Autodesk Inventor part; units mm, degrees
ref_plane "YZ Plane" through (0, 0, 0) normal (1, 0, 0) x (0, 1, 0)
ref_plane "XZ Plane" through (0, 0, 0) normal (0, 1, 0) x (-1, 0, 0)
ref_plane "XY Plane" through (0, 0, 0) normal (0, 0, 1) x (1, 0, 0)
sketch "草圖1" plane through (0, 0, 0) normal (0, 1, 0) x (-1, 0, 0)
  line L0 (0, 0) -> (60, 0)
  line L1 (60, 0) -> (60, -90)
  line L2 (60, -90) -> (0, -90)
  line L3 (0, -90) -> (0, 0)
  dimension "d0" = 60
  dimension "d1" = 90
extrude "擠出1" add sketch "草圖1" along normal blind 10
chamfer "倒角1" distance 5 angle 45 4 edges at (-60, 10, -45) (-30, 10, 0) (0, 10, -45) (-30, 10, -90)
sketch "草圖2" plane through (0, 10, 0) normal (0, 1, 0) x (1, 0, 0)
  line L0 (-60, 0) -> (0, 0)
  line L1 (0, 0) -> (-15, 0)
  line L2 (-15, 0) -> (-15, 10)
  line L3 (-15, 10) -> (0, 10)
  line L4 (0, 10) -> (0, 0)
  line L5 (-15, 10) -> (-30, 10)
  line L6 (-30, 10) -> (-30, 15)
  line L7 (-30, 15) -> (-15, 15)
  line L8 (-15, 15) -> (-15, 10)
  line L9 (-30, 15) -> (-35, 15)
  line L10 (-35, 15) -> (-35, 35)
  line L11 (-35, 35) -> (-30, 35)
  line L12 (-30, 35) -> (-30, 15)
  line L13 (-35, 35) -> (-50, 35)
  line L14 (-50, 35) -> (-50, 80)
  line L15 (-50, 80) -> (-35, 80)
  line L16 (-35, 80) -> (-35, 35)
  line L17 (-35, 80) -> (-20, 80)
  line L18 (-20, 80) -> (-20, 75)
  line L19 (-20, 75) -> (-35, 75)
  line L20 (-35, 75) -> (-35, 80)
  line L21 (-20, 75) -> (-10, 75)
  line L22 (-10, 75) -> (-10, 45)
  line L23 (-10, 45) -> (-20, 45)
  line L24 (-20, 45) -> (-20, 75)
  circle A0 centre (-15, 10) radius 3
  circle A1 centre (-30, 15) radius 3
  circle A2 centre (-35, 35) radius 3
  circle A3 centre (-50, 80) radius 3
  circle A4 centre (-20, 75) radius 3
  circle A5 centre (-10, 45) radius 3
  dimension "d7" = 15
  dimension "d8" = 10
  dimension "d9" = 15
  dimension "d10" = 5
  dimension "d11" = 5
  dimension "d12" = 20
  dimension "d13" = 15
  dimension "d14" = 45
  dimension "d15" = 15
  dimension "d16" = 5
  dimension "d17" = 10
  dimension "d18" = 30
  dimension "d19" = 6
  dimension "d20" = 6
  dimension "d21" = 6
  dimension "d22" = 6
  dimension "d23" = 6
  dimension "d24" = 6
extrude "擠出2" add sketch "草圖2" along normal blind 40 contours A5 L22 L23 | L23 L22 A5
extrude "擠出3" add sketch "草圖2" along normal blind 5 contours A4 L18 L19 | L19 L24 A4 | L18 A4 L21 | L21 A4 L24
extrude "擠出4" add sketch "草圖2" along normal blind 10 contours A3 L15 L14 | L14 L15 A3
extrude "擠出5" add sketch "草圖2" along normal blind 25 contours A2 L13 L10 | L10 L11 A2 | L11 L16 A2 | L13 A2 L16
extrude "擠出6" add sketch "草圖2" along normal blind 20 contours A0 L5 L2 | L2 L3 A0 | L8 A0 L3 | L5 A0 L8
extrude "擠出7" add sketch "草圖2" along normal blind 30 contours A1 L9 L6 | L6 L7 A1 | L7 L12 A1 | L9 A1 L12
sketch "草圖3" plane through (-15, 30, -10) normal (0, 1, 0) x (1, 0, 0)
  circle A0 centre (0, 0) radius 1.5
  point P0 (15, -10)
  dimension "d37" = 3
sketch "草圖4" plane through (-30, 40, -15) normal (0, 1, 0) x (1, 0, 0)
  circle A0 centre (0, 0) radius 1.5
  point P0 (30, -15)
  dimension "d38" = 3
sketch "草圖5" plane through (-10, 50, -45) normal (0, 1, 0) x (1, 0, 0)
  circle A0 centre (0, 0) radius 1.5
  point P0 (10, -45)
  dimension "d39" = 3
sketch "草圖6" plane through (-35, 35, -35) normal (0, 1, 0) x (1, 0, 0)
  circle A0 centre (0, 0) radius 1.5
  point P0 (35, -35)
  dimension "d40" = 3
sketch "草圖7" plane through (-50, 20, -80) normal (0, 1, 0) x (1, 0, 0)
  circle A0 centre (0, 0) radius 1.5
  point P0 (50, -80)
  dimension "d41" = 3
sketch "草圖8" plane through (-20, 15, -75) normal (0, 1, 0) x (1, 0, 0)
  circle A0 centre (0, 0) radius 1.5
  point P0 (20, -75)
  dimension "d42" = 3
extrude "擠出8" add sketch "草圖8" along normal blind 8
extrude "擠出9" add sketch "草圖5" along normal blind 8
extrude "擠出10" add sketch "草圖3" along normal blind 8
extrude "擠出11" add sketch "草圖4" along normal blind 8
extrude "擠出12" add sketch "草圖6" along normal blind 8
extrude "擠出13" add sketch "草圖7" along normal blind 8
chamfer "倒角2" distance 0.5 distance2 8 1 edges at (-51.5, 28, -80) measured on face at (-50.167, 28, -80.5524)
chamfer "倒角3" distance 0.5 distance2 8 1 edges at (-21.5, 23, -75) measured on face at (-20.167, 23, -75.5524)
chamfer "倒角4" distance 0.5 distance2 8 1 edges at (-11.5, 58, -45) measured on face at (-9.1644, 58, -45.3876)
chamfer "倒角5" distance 0.5 distance2 8 1 edges at (-36.5, 43, -35) measured on face at (-34.1644, 43, -35.3876)
chamfer "倒角6" distance 0.5 distance2 8 1 edges at (-31.5, 48, -15) measured on face at (-29.1644, 48, -15.3876)
chamfer "倒角7" distance 0.5 distance2 8 1 edges at (-16.5, 38, -10) measured on face at (-14.6048, 38, -9.3766)
properties part number "HeadTrackerProMax"
Here's how the part is built. I have some questions about the finished solid (model axes, mm). A direction names the side the tool comes from. Round coordinates to 2 decimals unless told otherwise and drop trailing zeros. Write each loop counter-clockwise with the first axis right and the second up, starting at its lowest first coordinate (ties: lowest second). Pieces come first, ordered by that corner, then holes.
Q1. If we section it at C-C on y = 36: Write out the boundary of the cut face in (x, z).
Q2. Will these pins go through, and if not, where does the flat tip stop? P1, Ø10, axis at y = 30, z = -31, coming from the +X side; P2, Ø5, axis at x = -14, z = -9, coming from the +Y side; P3, Ø1.8, axis at x = -29, z = -14, coming from the +Y side; P4, Ø8, axis at x = -51.5, z = -18, coming from the -Y side.
Q3. If we section it at D-D on y = 47: Write out the boundary of the cut face in (x, z), plus the area to 3 significant figures.
Q4. Please list where these lines run through material, in increasing order: probe 1 along Y at (x, z) = (-53, -55.5); probe 2 along X at (y, z) = (5.5, -50); probe 3 along Z at (x, y) = (-19, 18).
Q5. Which directions (+Z, -Z, +X, -X, +Y, -Y) give clear straight access to the entire face, cutting with the end or side of a thin tool? Please do faces 1 (the cylindrical face through (-52.4, 14.9, -81.8)), 2 (the flat face through (-50, 28, -80)).
Answer below:
1. outline: circle Ø2.88 at (-35, -35); circle Ø6 at (-30, -15); circle Ø2.25 at (-15, -10); circle Ø6 at (-10, -45)
2. P1: stops at x = -32
2. P2: stops at y = 38
2. P3: stops at y = 48
2. P4: stops at y = 0
3. outline: circle Ø2.13 at (-30, -15); circle Ø6 at (-10, -45)
3. area: 31.8 mm2
4. probe 1: y = 0 to 10
4. probe 2: x = -59.5 to -0.5
4. probe 3: z = -75.85 to -74.15
5. face 1: +Y
5. face 2: +Z, -Z, +X, -X, +Y
